Could you check a few things on this model? Use its own coordinates, in mm. Give positions to 0.01 mm unless a question says otherwise; leave off trailing zeros. Loops run counter-clockwise (first coordinate to the right, second up) from the corner with the lowest first, then second, coordinate; pieces in that order, holes last. Notation, with made-up numbers: (-21, 87.25) -> (7, 87.25) arc R19 ccw to (7, 108.25) -> close; hole circle Ø1 at (31.25, -16.5). An arc over 180 degrees is marked (long way). Put each result on its own line as item: value.
```python
from build123d import *

# Parameters (mm, degrees)
F1_DEPTH = 10
F5_DEPTH = 10
F6_DEPTH = 10
F7_DEPTH = 10


with BuildPart() as f1:
    # F0 (on Top) → F1 (new body)
    with BuildSketch(Plane.XY):
        with BuildLine():
            Line((744, 273.5), (-744, 273.5))
            ThreePointArc((-744, 273.5), (-765.213203, 264.713203), (-774, 243.5))
            Line((-774, 243.5), (-774, -243.5))
            ThreePointArc((-774, -243.5), (-765.213203, -264.713203), (-744, -273.5))
            Line((-744, -273.5), (744, -273.5))
            ThreePointArc((744, -273.5), (765.213203, -264.713203), (774, -243.5))
            Line((774, -243.5), (774, 243.5))
            ThreePointArc((774, 243.5), (765.213203, 264.713203), (744, 273.5))
        make_face()
    extrude(amount=-F1_DEPTH)

    # F2 (on face) → F5 (join)
    with BuildSketch(Plane.XY):
        with BuildLine():
            Line((237.563882, 186.23467), (237.563882, -243.76533))
            Line((237.563882, -243.76533), (737.563882, -243.76533))
            ThreePointArc((737.563882, -243.76533), (744.63495, -240.836398), (747.563882, -233.76533))
            Line((747.563882, -233.76533), (747.563882, 186.23467))
            ThreePointArc((747.563882, 186.23467), (744.63495, 193.305738), (737.563882, 196.23467))
            Line((737.563882, 196.23467), (247.563882, 196.23467))
            ThreePointArc((247.563882, 196.23467), (240.492814, 193.305738), (237.563882, 186.23467))
        make_face()
    extrude(amount=F5_DEPTH)

    # F3 (on face) → F6 (join)
    with BuildSketch(Plane.XY):
        with BuildLine():
            Line((-441.157219, 201.522775), (-721.157219, 201.522775))
            ThreePointArc((-721.157219, 201.522775), (-728.228287, 198.593843), (-731.157219, 191.522775))
            Line((-731.157219, 191.522775), (-731.157219, -238.477225))
            ThreePointArc((-731.157219, -238.477225), (-728.228287, -245.548292), (-721.157219, -248.477225))
            Line((-721.157219, -248.477225), (-441.157219, -248.477225))
            ThreePointArc((-441.157219, -248.477225), (-434.086152, -245.548292), (-431.157219, -238.477225))
            Line((-431.157219, -238.477225), (-431.157219, 191.522775))
            ThreePointArc((-431.157219, 191.522775), (-434.086152, 198.593843), (-441.157219, 201.522775))
        make_face()
    extrude(amount=F6_DEPTH)

    # F4 (on face) → F7 (join)
    with BuildSketch(Plane.XY):
        with BuildLine():
            Line((43.649018, 52.653256), (-261.350982, 52.653256))
            ThreePointArc((-261.350982, 52.653256), (-268.42205, 49.724324), (-271.350982, 42.653256))
            Line((-271.350982, 42.653256), (-271.350982, -237.346744))
            ThreePointArc((-271.350982, -237.346744), (-268.42205, -244.417812), (-261.350982, -247.346744))
            Line((-261.350982, -247.346744), (43.649018, -247.346744))
            ThreePointArc((43.649018, -247.346744), (50.720086, -244.417812), (53.649018, -237.346744))
            Line((53.649018, -237.346744), (53.649018, 42.653256))
            ThreePointArc((53.649018, 42.653256), (50.720086, 49.724324), (43.649018, 52.653256))
        make_face()
    extrude(amount=F7_DEPTH)


solid = f1.part
```
1. If we section it at C-C (y = 130): List the corners of the cut face in (x, z) for me.
Recorded:
outline: (-774, -10) -> (774, -10) -> (774, 0) -> (747.56, 0) -> (747.56, 10) -> (237.56, 10) -> (237.56, 0) -> (-431.16, 0) -> (-431.16, 10) -> (-731.16, 10) -> (-731.16, 0) -> (-774, 0) -> close
2. If we section it at D-D (y = -167): List the corners of the cut face in (x, z) for me, then the cut area to 3 significant figures.
Recorded:
outline: (-774, -10) -> (774, -10) -> (774, 0) -> (747.56, 0) -> (747.56, 10) -> (237.56, 10) -> (237.56, 0) -> (53.65, 0) -> (53.65, 10) -> (-271.35, 10) -> (-271.35, 0) -> (-431.16, 0) -> (-431.16, 10) -> (-731.16, 10) -> (-731.16, 0) -> (-774, 0) -> close
area: 26,800 mm^2
3. I'm going to push flat-ended pins straight in: pin 1 (11 mm diameter, centred on y = -80, z = 7.5, fed in from -X); pin 2 (3 mm diameter, centred on x = -601, z = 5.5, fed in from -Y); pin 3 (1 mm diameter, centred on y = -127, z = 2, fed in from +X); pin 4 (10 mm diameter, centred on x = -276.5, z = 2.5, fed in from +Y). Where does each tip first touch, or does it pass through?
Recorded:
pin 1: stops at x = -731.16
pin 2: stops at y = -248.48
pin 3: stops at x = 747.56
pin 4: stops at y = 273.5
4. If we section it at B-B (x = -192.5): List the corners of the cut face in (y, z) for me, then the cut area to 3 significant figures.
Recorded:
outline: (-273.5, -10) -> (273.5, -10) -> (273.5, 0) -> (52.65, 0) -> (52.65, 10) -> (-247.35, 10) -> (-247.35, 0) -> (-273.5, 0) -> close
area: 8,470 mm^2
5. If we section it at A-A (z = 5.25): List the corners of the cut face in (x, y) for me.
Recorded:
outline: (-731.16, -238.48) arc R10 ccw to (-721.16, -248.48) -> (-441.16, -248.48) arc R10 ccw to (-431.16, -238.48) -> (-431.16, 191.52) arc R10 ccw to (-441.16, 201.52) -> (-721.16, 201.52) arc R10 ccw to (-731.16, 191.52) -> close; (-271.35, -237.35) arc R10 ccw to (-261.35, -247.35) -> (43.65, -247.35) arc R10 ccw to (53.65, -237.35) -> (53.65, 42.65) arc R10 ccw to (43.65, 52.65) -> (-261.35, 52.65) arc R10 ccw to (-271.35, 42.65) -> close; (237.56, -243.77) -> (737.56, -243.77) arc R10 ccw to (747.56, -233.77) -> (747.56, 186.23) arc R10 ccw to (737.56, 196.23) -> (247.56, 196.23) arc R10 ccw to (237.56, 186.23) -> close
6. I need wall thicknesses on line 1 (X direction, y = 137, z = 2.25); line 2 (Y direction, x = 410, z = 5); line 3 (Y direction, x = -686, z = 3.5). Which ranges of each line are inside material? Lowest first, please.
Recorded:
line 1: x = -731.16 to -431.16, 237.56 to 747.56
line 2: y = -243.77 to 196.23
line 3: y = -248.48 to 201.52
